CAD build for the part. Positions are in the model's coordinates, mm. A direction names the side the tool comes from. Give positions to 0.01 mm unless a question says otherwise; leave off trailing zeros. Loops run counter-clockwise (first coordinate to the right, second up) from the corner with the lowest first, then second, coordinate; pieces in that order, holes last.
```python
from build123d import *

# Parameters (mm, degrees)
SKETCH_1_W          = 52
SKETCH_1_H          = 30
EXTRUDE_1_DEPTH     = 3
SKETCH_2_W          = 3
SKETCH_2_H          = 5
CUT_EXTRUDE_1_DEPTH = 4
SKETCH_6_W          = 4.623864405
SKETCH_6_H          = 6.377744006
EXTRUDE_2_DEPTH     = 3
SKETCH_7_W          = 3
SKETCH_7_H          = 5
CUT_EXTRUDE_4_DEPTH = 10
SKETCH_9_R          = 2
EXTRUDE_3_DEPTH     = 3
SKETCH_10_R         = 2.25
CUT_EXTRUDE_5_DEPTH = 10
SKETCH_11_R         = 1.5
CUT_EXTRUDE_6_DEPTH = 10
SKETCH_12_R         = 11
CUT_EXTRUDE_7_DEPTH = 10
FILLET_1_R          = 2
SKETCH_13_W         = 2
SKETCH_13_H         = 36.695
EXTRUDE_4_DEPTH     = 3
FILLET_2_R          = 2
CHAMFER_1_SIZE      = 7
CHAMFER_1_SIZE2     = 15.011548444
FILLET_3_R          = 2
SKETCH_15_R         = 2.25
SKETCH_15_R_2       = 2.15
EXTRUDE_6_DEPTH     = 3
FILLET_4_R          = 2


with BuildPart() as part:
    # 草图1 → 凸台-拉伸1 (new body)
    with BuildSketch(Plane.XY):
        Rectangle(SKETCH_1_W, SKETCH_1_H)
    extrude(amount=EXTRUDE_1_DEPTH)

    # 草图2 → 切除-拉伸1 (cut)
    with BuildSketch(Plane.XY.offset(3)):
        with Locations((22, -7.5)):
            Rectangle(SKETCH_2_W, SKETCH_2_H)
        with Locations((22, 9.5)):
            Rectangle(SKETCH_2_W, SKETCH_2_H)
        with Locations((-22, 9.5)):
            Rectangle(SKETCH_2_W, SKETCH_2_H)
        with Locations((-22, -7.5)):
            Rectangle(SKETCH_2_W, SKETCH_2_H)
    extrude(amount=-CUT_EXTRUDE_1_DEPTH, mode=Mode.SUBTRACT)

    # 草图6 → 凸台-拉伸2 (add)
    with BuildSketch(Plane(origin=(0, 0, 0), x_dir=(-1, 0, 0), z_dir=(0, 0, -1))):
        with Locations((-21.865764725, 9.519388139)):
            Rectangle(SKETCH_6_W, SKETCH_6_H)
    extrude(amount=-EXTRUDE_2_DEPTH)

    # 草图7 → 切除-拉伸4 (cut)
    with BuildSketch(Plane(origin=(0, 0, 0), x_dir=(-1, 0, 0), z_dir=(0, 0, -1))):
        with Locations((-22, 3.5)):
            Rectangle(SKETCH_7_W, SKETCH_7_H)
    extrude(amount=-CUT_EXTRUDE_4_DEPTH, mode=Mode.SUBTRACT)

    # 草图9 → 凸台-拉伸3 (add)
    with BuildSketch(Plane.XY.offset(3)):
        Polygon((26, 15), (31.495, 15), (31.495, -21.695), (20.5, -21.695), (20.5, -15), (26, -15), align=None)
        with Locations((27.995, -16.195)):
            Circle(SKETCH_9_R, mode=Mode.SUBTRACT)
    extrude(amount=-EXTRUDE_3_DEPTH)

    # 草图10 → 切除-拉伸5 (cut)
    with BuildSketch(Plane.XY.offset(3)):
        with Locations((27.995, -16.195)):
            Circle(SKETCH_10_R)
    extrude(amount=-CUT_EXTRUDE_5_DEPTH, mode=Mode.SUBTRACT)

    # 草图11 → 切除-拉伸6 (cut)
    with BuildSketch(Plane.XY.offset(3)):
        with Locations((2.5, -3)):
            Circle(SKETCH_11_R)
        with Locations((16.5, -3)):
            Circle(SKETCH_11_R)
        with Locations((9.5, -10)):
            Circle(SKETCH_11_R)
    extrude(amount=-CUT_EXTRUDE_6_DEPTH, mode=Mode.SUBTRACT)

    # 草图12 → 切除-拉伸7 (cut)
    with BuildSketch(Plane.XY.offset(3)):
        with Locations((9.5, 17.5)):
            Circle(SKETCH_12_R)
    extrude(amount=-CUT_EXTRUDE_7_DEPTH, mode=Mode.SUBTRACT)

    # 圆角1
    fillet_1_edges = [part.edges().sort_by_distance(p)[0] for p in [
        (20.5, -15, 1.5),
        (20.212142643, 15, 1.5),
        (-1.212142643, 15, 1.5),
    ]]
    fillet(fillet_1_edges, radius=FILLET_1_R)

    # 草图13 → 凸台-拉伸4 (add)
    with BuildSketch(Plane.XY.offset(3)):
        with Locations((32.495, -3.3475)):
            Rectangle(SKETCH_13_W, SKETCH_13_H)
    extrude(amount=-EXTRUDE_4_DEPTH)

    # 圆角2
    fillet_2_edges = [part.edges().sort_by_distance(p)[0] for p in [
        (33.495, -21.695, 1.5),
    ]]
    fillet(fillet_2_edges, radius=FILLET_2_R)

    # 倒角1
    chamfer_1_edges = [part.edges().sort_by_distance(p)[0] for p in [
        (33.495, 15, 1.5),
    ]]
    chamfer_1_side = [part.faces().sort_by_distance(p)[0] for p in [
        (27.595655459, 15, 1.5),
    ]]
    chamfer(chamfer_1_edges, length=CHAMFER_1_SIZE, length2=CHAMFER_1_SIZE2, reference=chamfer_1_side[0])

    # 圆角3
    fillet_3_edges = [part.edges().sort_by_distance(p)[0] for p in [
        (33.495, -0.011548444, 1.5),
        (26.495, 15, 1.5),
    ]]
    fillet(fillet_3_edges, radius=FILLET_3_R)

    # 草图15 → 凸台-拉伸6 (add)
    with BuildSketch(Plane.XY.offset(3)):
        with Locations((27.995, -16.195)):
            Circle(SKETCH_15_R)
        with Locations((27.995, -16.195)):
            Circle(SKETCH_15_R_2, mode=Mode.SUBTRACT)
    extrude(amount=-EXTRUDE_6_DEPTH)

    # 圆角4
    fillet_4_edges = [part.edges().sort_by_distance(p)[0] for p in [
        (-26, -15, 1.5),
        (-26, 15, 1.5),
    ]]
    fillet(fillet_4_edges, radius=FILLET_4_R)


solid = part.part
```
1. Saw through at C-C, the plane x = 2.5. List the corners of the cut face in (y, z).
Responses:
outline: (-15, 0) - (-4.5, 0) - (-4.5, 3) - (-15, 3) - close; (-1.5, 0) - (9.01, 0) - (9.01, 3) - (-1.5, 3) - close
2. Pull direction X, two halves, no side cores. Call faces 1 (the face through (3, 1, 3)), 2 (the face through (20.567, 14.651, 1.521)), 3 (the face through (-25.4, -14.43, 1.52)): released by +X, released by -X, zero draft, split by the parting line, or undercut.
Responses:
face 1: zero draft
face 2: undercut
face 3: released by -X
3. Saw through at B-B, the plane y = -3. List the corners of the cut face in (x, z) (3 decimals).
Responses:
outline: (-26, 0) - (1, 0) - (1, 3) - (-26, 3) - close; (4, 0) - (15, 0) - (15, 3) - (4, 3) - close; (18, 0) - (33.495, 0) - (33.495, 3) - (18, 3) - close
4. Saw through at A-A, the plane x = -22. List the corners of the cut face in (y, z).
Responses:
outline: (-15, 0) - (-10, 0) - (-10, 3) - (-15, 3) - close; (-5, 0) - (7, 0) - (7, 3) - (-5, 3) - close; (12, 0) - (15, 0) - (15, 3) - (12, 3) - close
5. Probe line 1 along X through (y, z) = (-6, 0.7) (3 decimals); line 2 along Y through (x, z) = (2.5, 2); line 3 along Y through (x, z) = (27.5, 0.8) (3 decimals). List the from-to ranges inside material, lowest first.
Responses:
line 1: x = -26 to -23.5, -20.5 to 20.5, 23.5 to 33.495
line 2: y = -15 to -4.5, -1.5 to 9.01
line 3: y = -21.695 to -18.287, -14.103 to 12.845
6. Tool access for faces 4 (the face through (-23.5, 9, 2)), 5 (the face through (-1.54, 14.63, 1.52)), 6 (the face through (26, -21.695, 2)): list every direction of +Z, -Z, +X, -X, +Y, -Y with a clear straight run to the whole face (end or side of a thin tool).
Responses:
face 4: +Z, -Z
face 5: +Z, -Z, +Y
face 6: +Z, -Z, +X, -X, -Y
7. Drop a flat-ended pin along its axis: pin 1 (1.8 mm diameter, centred on x = 2.5, y = -3, fed in from +Z). Give the stop position or say it passes through.
Responses:
pin 1: passes through
8. Saw through at D-D, the plane z = 1.7. Count the separate pieces of the cut face and the enclosed holes in it, and give its area (3 significant figures).
Responses:
separate pieces: 1
enclosed holes: 8
area: 1,590 mm2
